Work out the finished part from the listing and answer in its coordinate system (mm). Face numbers are marked on the shaded views. Coordinates: 2 decimals unless noted, no trailing zeros. Loops run counter-clockwise (first coordinate to the right, second up) from the corner with the lowest first, then second, coordinate; pieces in that order, holes last. Notation, with made-up numbers: (-18.75, 81) -> (-2.75, 81) arc R27 ccw to (-2.75, 100) -> close; hole circle Ø10 at (18, -24.5). An arc over 180 degrees is marked (long way). One line per question, with ' | ' between items.
Autodesk Inventor part; units mm, degrees
ref_plane "YZ Plane" through (0, 0, 0) normal (1, 0, 0) x (0, 1, 0)
ref_plane "XZ Plane" through (0, 0, 0) normal (0, 1, 0) x (-1, 0, 0)
ref_plane "XY Plane" through (0, 0, 0) normal (0, 0, 1) x (1, 0, 0)
sketch "Skizze1" plane through (0, 0, 0) normal (0, 0, 1) x (1, 0, 0)
  circle A0 centre (0, 0) radius 3.1
  circle A1 centre (0, 0) radius 7.5
  dimension "d0" = 6.2
  dimension "d1" = 15
extrude "Extrusion1" add sketch "Skizze1" along normal blind 12
extrude "Extrusion2" add sketch "Skizze1" against normal blind 3 contours A0 | A1
fillet "Rundung1" radius 1 1 edges at (-7.5, 0, -3)
properties part number "Knopf"
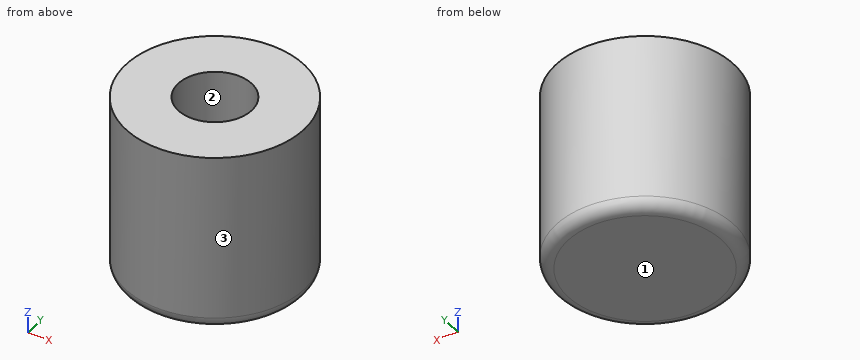
1) Find section D-D (z = -1.5). Write down the section's boundary in (x, y).
Check values:
outline: circle Ø15 at (0, 0)
2) Find the intervals of material crossed by line 1 along Y through (x, z) = (0, 9.25); line 2 along Z through (x, y) = (0, -0.75); line 3 along X through (y, z) = (2.25, 9), in increasing order.
Check values:
line 1: y = -7.5 to -3.1, 3.1 to 7.5 | line 2: z = -3 to 0 | line 3: x = -7.15 to -2.13, 2.13 to 7.15
3) Find section C-C (z = 6.5). Write down the section's boundary in (x, y), plus the area to 3 significant figures.
Check values:
outline: circle Ø15 at (0, 0); hole circle Ø6.2 at (0, 0) | area: 147 mm^2
4) Find section A-A (x = 0). Write down the section's boundary in (y, z).
Check values:
outline: (-7.5, -2) arc R1 ccw to (-6.5, -3) -> (6.5, -3) arc R1 ccw to (7.5, -2) -> (7.5, 12) -> (3.1, 12) -> (3.1, 0) -> (-3.1, 0) -> (-3.1, 12) -> (-7.5, 12) -> close
5) Flat-ended cylindrical pins translate along their axes: pin 1 (2 mm diameter, centred on x = -4, z = 7, fed in from -Y); pin 2 (3 mm diameter, centred on y = 2.5, z = 8.5, fed in from +X); pin 3 (4 mm diameter, centred on y = 5.5, z = 9, fed in from -X); pin 4 (8 mm diameter, centred on y = -0.5, z = -1, fed in from +X). Find the tip coordinate at first contact, or state that the pin passes through.
Check values:
pin 1: stops at y = -6.87 | pin 2: stops at x = 7.43 | pin 3: stops at x = -6.63 | pin 4: stops at x = 7.5
6) The mould has two halves that part along X. Classify the marked faces 1, 2 and 3: released by +X, released by -X, zero draft, split by the parting line, or undercut.
Check values:
face 1: zero draft | face 2: undercut | face 3: split by the parting line
